```python
from build123d import *

# Parameters (mm, degrees)
F1_DEPTH = 63.5
F0_W     = 25.4
F0_H     = 19.0499988828
F2_DEPTH = 25.4
F3_DEPTH = 7.9375
F0_H_2   = 4.7498011172
F5_R     = 6.35


with BuildPart() as f1:
    # F0 (on Front) → F1 (new body, symmetric)
    with BuildSketch(Plane.XZ):
        Polygon((-41.275, -9.525), (41.275, -9.525), (41.275, 9.525), (22.2250011172, 9.525), (-41.275, 9.525), align=None)
    extrude(amount=F1_DEPTH, both=True)

    # F0 (on Front) → F2 (join, symmetric)
    with BuildSketch(Plane.XZ):
        with BuildLine():
            Line((22.2250011172, 9.525), (41.275, 9.525))
            Line((41.275, 9.525), (41.275, 27.0012465922))
            ThreePointArc((41.275, 27.0012465922), (45.989313778, 38.2908306436), (57.332286054, 42.8752))
            Line((57.332286054, 42.8752), (60.325, 42.8752))
            Line((60.325, 42.8752), (60.325, 61.9251988828))
            Line((60.325, 61.9251988828), (57.420376338, 61.9251988828))
            add(Edge.make_bspline(
                [(55.8653542089, 61.902610923), (56.3842660516, 61.9141182995), (56.9026324706, 61.9216689247), (57.420376338, 61.9251988828)],
                knots=[110.5091164391, 110.5091164391, 110.5091164391, 110.5091164391, 111.7432689403, 111.7432689403, 111.7432689403, 111.7432689403], degree=3))
            ThreePointArc((55.8653542089, 61.902610923), (32.0042071135, 51.2385040086), (22.2250011172, 27.0012465922))
            Line((22.2250011172, 27.0012465922), (22.2250011172, 9.525))
        make_face()
        with Locations((73.025, 52.4001994414)):
            Rectangle(F0_W, F0_H)
    extrude(amount=F2_DEPTH, both=True)

    # F0 (on Front) → F3 (join, symmetric)
    with BuildSketch(Plane.XZ):
        with BuildLine():
            add(Edge.make_bspline(
                [(-41.275, 9.525), (-41.4371192088, 28.1171277164), (9.4006837592, 60.8722115153), (55.8653542089, 61.902610923)],
                knots=[0, 0, 0, 0, 110.5091164391, 110.5091164391, 110.5091164391, 110.5091164391], degree=3))
            Line((-41.275, 9.525), (22.2250011172, 9.525))
            Line((22.2250011172, 9.525), (22.2250011172, 27.0012465922))
            ThreePointArc((22.2250011172, 27.0012465922), (32.0042071135, 51.2385040086), (55.8653542089, 61.902610923))
        make_face()
    extrude(amount=F3_DEPTH, both=True)

    # F0 (on Front) → F4 (revolve)
    with BuildSketch(Plane.XZ):
        with Locations((98.425, 64.3000994414)):
            Rectangle(F0_W, F0_H_2)
        Polygon((85.725, 61.9251988828), (85.725, 42.8752), (85.725, 38.1), (111.125, 38.1), (111.125, 61.9251988828), align=None)
    revolve(axis=Axis((85.725, 0, 52.3875), (0, 0, 1)))

    # F5
    f5_edges = [f1.edges().sort_by_distance(p)[0] for p in [
        (-41.275, -63.5, 0),
        (41.275, -63.5, 0),
        (41.275, 63.5, 0),
        (-41.275, 63.5, 0),
    ]]
    fillet(f5_edges, radius=F5_R)


solid = f1.part
```
The listing builds one solid part. Answer for the finished solid, in the listing's coordinates (mm). A direction names the side the tool comes from. Give positions to 0.01 mm unless a question says otherwise; leave off trailing zeros. Order: outer loops, then holes, each group sorted by start corner. A loop starts at its lowest first (then second) coordinate and runs counter-clockwise, first axis right, second up. Notation, with made-up numbers: (47.5, 85.5) -> (67.5, 85.5) arc R25 ccw to (67.5, 122.5) -> close; hole circle Ø11 at (83, 11). An arc over 180 degrees is marked (long way). Answer as a JSON object with one key per item and string values. Group by question number.
Item 1: A tool of negligible diameter and unlimited length cuts with its end or side. For faces 1 (the flat face through (46, 25.4, 42)), 2 (the flat face through (-3, 7.938, 30)), 3 (the flat face through (1, -36, 9.525)), from which of +Z, -Z, +X, -X, +Y, -Y can it reach the whole face along a straight path? Write none if from no direction.
Item 2: Determine the mould class of faces 4 (the flat face through (41.275, -1, 4)), 5 (the flat face through (60, 0, 61.925)), 6 (the cylindrical face through (45.9, -0.4, 38.2)) for opening direction X: pulls with the +X half, pulls with the -X half, needs draft (parallel to the pull), parting line crosses it, or undercut.
Item 3: The part is cut by section A-A on z = -3. Write down the section's boundary in (x, y) (3 decimals).
Item 4: Flat-ended cylindrical pins translate along their axes: pin 1 (14 mm diameter, centred on x = 76, y = 8, fed in from -Z); pin 2 (15.5 mm diameter, centred on x = 31.5, z = 39.5, fed in from -Y); pin 3 (10 mm diameter, centred on y = 10.5, z = 38, fed in from -X). Find the tip coordinate at first contact, or state that the pin passes through.
Item 5: Consider L1, parallel to Y at x = 33, z = 25; L2, parallel to X at y = 46.5, z = 1 (3 decimals); L3, parallel to Y at x = -19, z = 34.5. Determine where each line is inside the solid, lowest interval first. Write a range as from..to.
Item 6: The part is cut by section B-B on x = 78. Write down the section's boundary in (y, z) (3 decimals), and give its area (3 significant figures).
Result set:
{
 "1": {"face 1": "+Z, +X, -X, +Y", "face 2": "+Z, -X, +Y", "face 3": "+Z, -X, -Y"},
 "2": {"face 4": "pulls with the +X half", "face 5": "needs draft", "face 6": "undercut"},
 "3": {"outline": "(-41.275, -57.15) arc R6.35 ccw to (-34.925, -63.5) -> (34.925, -63.5) arc R6.35 ccw to (41.275, -57.15) -> (41.275, 57.15) arc R6.35 ccw to (34.925, 63.5) -> (-34.925, 63.5) arc R6.35 ccw to (-41.275, 57.15) -> close"},
 "4": {"pin 1": "z = 38.1", "pin 2": "y = -25.4", "pin 3": "x = -23.25"},
 "5": {"L1": "-25.4..25.4", "L2": "-41.275..41.275", "L3": "-7.94..7.94"},
 "6": {"outline": "(-25.4, 42.875) -> (-24.197, 42.875) -> (-24.197, 38.1) -> (24.197, 38.1) -> (24.197, 42.875) -> (25.4, 42.875) -> (25.4, 61.925) -> (24.197, 61.925) -> (24.197, 66.675) -> (-24.197, 66.675) -> (-24.197, 61.925) -> (-25.4, 61.925) -> close", "area": "1,430 mm²"}
}
